Check sheet for the modelled part. Datum: model origin and axes. Units: mm. Face numbers are marked on the shaded views. Give positions to 0.01 mm unless a question says otherwise; leave off trailing zeros. Loops run counter-clockwise (first coordinate to the right, second up) from the corner with the lowest first, then second, coordinate; pieces in that order, holes last. Notation, with made-up numbers: (46.5, 85.25) - (102.5, 85.25) arc R15 ccw to (102.5, 103.25) - close; hole circle Ø10 at (70.5, 73). An arc over 180 degrees is marked (long way). Answer in a Markdown table with one row per item. Add a question column.
(1) Sectioned sample at D-D on x = -12. Enter the section's corners in (y, z).
(2) Draft check along Z on the marked faces 1 and 2. Enter one of: released by +Z, released by -Z, zero draft, split by the parting line, or undercut.
(3) Thickness scan on L1, parallel to X at y = 1.15, z = 0; L2, parallel to X at y = 1.2, z = 0.75; L3, parallel to Z at x = 9.75, y = 1.5. Record the ranges inside material, lowest first.
(4) Sectioned sample at B-B on y = 1.2. Enter the section's corners in (x, z).
(5) Sectioned sample at A-A on x = 10. Enter the section's corners in (y, z).
(6) Sectioned sample at C-C on z = 0. Enter the section's corners in (x, y).
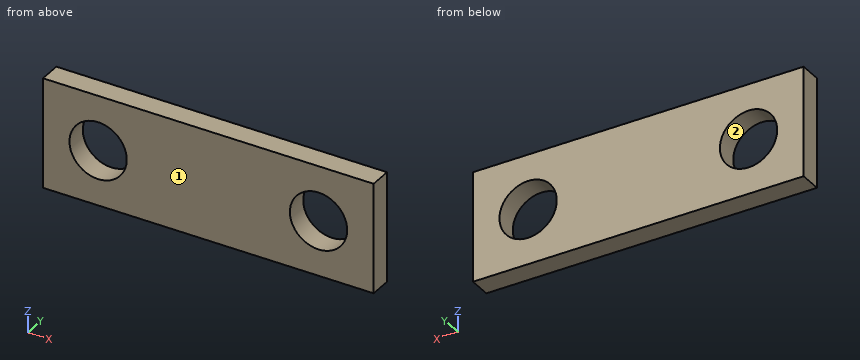
from build123d import *

# Parameters (mm, degrees)
SKETCH_1_W          = 30
SKETCH_1_H          = 10
EXTRUDE_1_DEPTH     = 2
SKETCH_2_R          = 2.6
CUT_EXTRUDE_1_DEPTH = 10


with BuildPart() as part:
    # 草图1 → 凸台-拉伸1 (new body)
    # profile 1 of 2: a face of its own
    with BuildSketch(Plane(origin=(0, 0, 0), x_dir=(1, 0, 0), z_dir=(0, 1, 0))):
        Rectangle(SKETCH_1_W, SKETCH_1_H)
        with BuildLine():
            Line((10, -2.5), (-10, -2.5))
            ThreePointArc((-10, -2.5), (-12.5, 0), (-10, 2.5))
            Line((-10, 2.5), (10, 2.5))
            ThreePointArc((10, 2.5), (11.767766953, 1.767766953), (12.5, 0))
            ThreePointArc((12.5, 0), (11.767766953, -1.767766953), (10, -2.5))
        make_face(mode=Mode.SUBTRACT)
    # profile 2 of 2: a face of its own
    with BuildSketch(Plane(origin=(0, 0, 0), x_dir=(1, 0, 0), z_dir=(0, 1, 0))):
        with BuildLine():
            ThreePointArc((-7.5, 0), (-8.232233047, -1.767766953), (-10, -2.5))
            Line((-10, -2.5), (10, -2.5))
            ThreePointArc((10, -2.5), (7.5, 0), (10, 2.5))
            Line((10, 2.5), (-10, 2.5))
            ThreePointArc((-10, 2.5), (-8.232233047, 1.767766953), (-7.5, 0))
        make_face()
    extrude(amount=EXTRUDE_1_DEPTH)

    # 草图2 → 切除-拉伸1 (cut)
    with BuildSketch(Plane.XZ):
        with Locations(Location((-10, 0, 0), (0, 0, 270))):
            Circle(SKETCH_2_R)
        with Locations(Location((10, 0, 0), (0, 0, 270))):
            Circle(SKETCH_2_R)
    extrude(amount=-CUT_EXTRUDE_1_DEPTH, mode=Mode.SUBTRACT)


solid = part.part
Reply:
| question | item | result |
|---|---|---|
| 1 | outline | (0, -5) - (2, -5) - (2, -1.66) - (0, -1.66) - close; (0, 1.66) - (2, 1.66) - (2, 5) - (0, 5) - close |
| 2 | face 1 | zero draft |
| 2 | face 2 | undercut |
| 3 | L1 | -15 to -12.6, -7.4 to 7.4, 12.6 to 15 |
| 3 | L2 | -15 to -12.49, -7.51 to 7.51, 12.49 to 15 |
| 3 | L3 | -5 to -2.59, 2.59 to 5 |
| 4 | outline | (-15, -5) - (15, -5) - (15, 5) - (-15, 5) - close; hole circle Ø5.2 at (-10, 0); hole circle Ø5.2 at (10, 0) |
| 5 | outline | (0, -5) - (2, -5) - (2, -2.6) - (0, -2.6) - close; (0, 2.6) - (2, 2.6) - (2, 5) - (0, 5) - close |
| 6 | outline | (-15, 0) - (-12.6, 0) - (-12.6, 2) - (-15, 2) - close; (-7.4, 0) - (7.4, 0) - (7.4, 2) - (-7.4, 2) - close; (12.6, 0) - (15, 0) - (15, 2) - (12.6, 2) - close |
